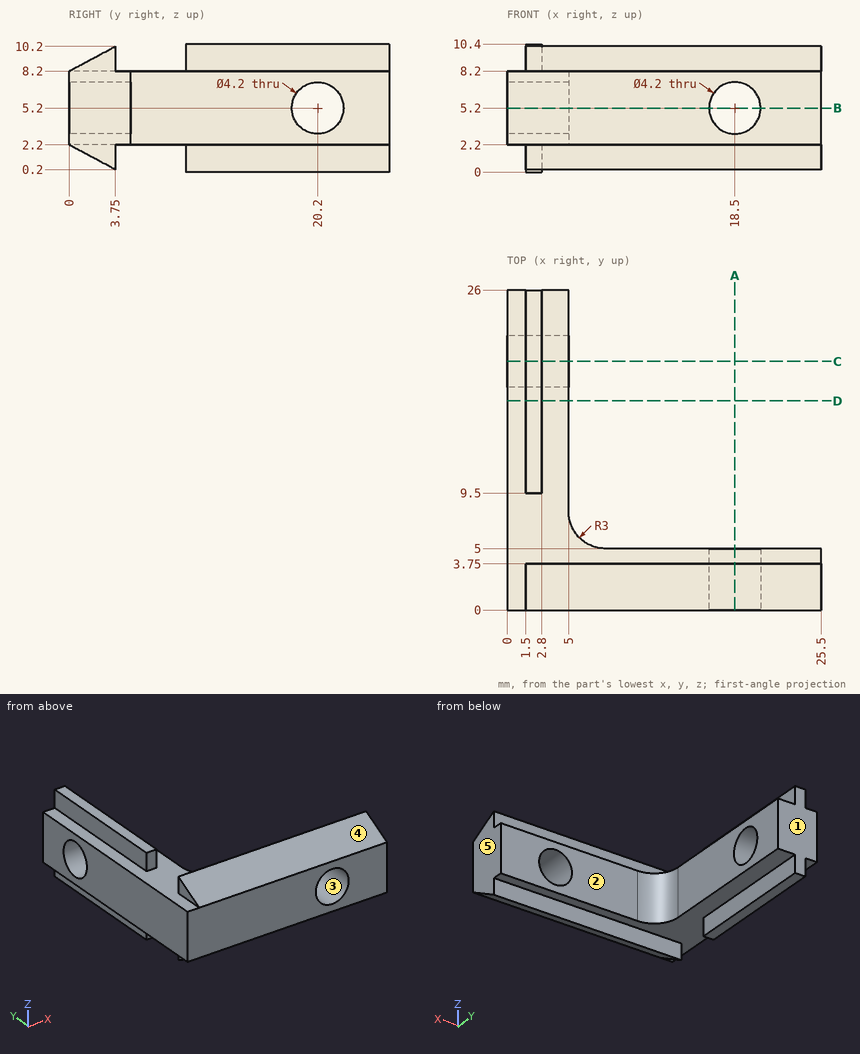
Study the drawing (mm; zero at the part's minimum x, y, z) and answer. A direction names the side the tool comes from. Coordinates: 2 decimals unless noted, no trailing zeros. Loops run counter-clockwise (first coordinate to the right, second up) from the corner with the lowest first, then second, coordinate; pieces in that order, holes last. Notation, with made-up numbers: (47.5, 27) -> (86.5, 27) arc R21 ccw to (86.5, 43) -> close; hole circle Ø8 at (0, -18.75). An arc over 180 degrees is marked (long way). Write each question's results on one line, items separated by ' | '. Start each with the question number.
1) For the marked faces 1 and 2, determine the directions among +Z, -Z, +X, -X, +Y, -Y from which every point of the face is accessible in a straight line to the end or side of a thin tool.
2) Find section D-D on y = 17. Determine the outline of the cut face in (x, z).
3) Find section A-A on x = 18.5. Determine the outline of the cut face in (y, z), then the cut area to 3 significant figures.
4) Consider line 1 along Z through (x, y) = (18.5, 3.9); line 2 along Y through (x, z) = (2.3, 5.2); line 3 along Z through (x, y) = (3.75, 11.25). Determine where each line is inside the solid, lowest interval first.
5) Find section C-C on y = 20.2. Determine the outline of the cut face in (x, z).
6) The mould has two halves that part along Z. Classify the marked faces 3, 4 and 5: pulls with the +Z half, pulls with the -Z half, needs draft (parallel to the pull), parting line crosses it, or undercut.
7) Flat-ended cylindrical pins translate along their axes: P1, Ø10, axis at x = 22.5, y = 6, coming from the -Z side; P2, Ø2.5, axis at y = 13.5, z = 0.5, coming from the +X side; P3, Ø2, axis at x = 6.5, z = 6.5, coming from the +Y side; P4, Ø3.5, axis at y = 20.2, z = 5.2, coming from the +X side. Find the tip coordinate at first contact, or state that the pin passes through.
8) Find section B-B on z = 5.2. Determine the outline of the cut face in (x, y).
Response values:
1) face 1: +Z, -Z, +X, -X, +Y | face 2: +Z, -Z, +X, +Y
2) outline: (0, 2.2) -> (1.5, 2.2) -> (1.5, 0) -> (2.8, 0) -> (2.8, 2.2) -> (5, 2.2) -> (5, 8.2) -> (2.8, 8.2) -> (2.8, 10.4) -> (1.5, 10.4) -> (1.5, 8.2) -> (0, 8.2) -> close
3) outline: (0, 2.2) -> (3.75, 0.2) -> (3.75, 2.2) -> (5, 2.2) -> (5, 3.1) -> (0, 3.1) -> close; (0, 7.3) -> (5, 7.3) -> (5, 8.2) -> (3.75, 8.2) -> (3.75, 10.2) -> (0, 8.2) -> close | area: 16.5 mm^2
4) line 1: z = 2.2 to 3.1, 7.3 to 8.2 | line 2: y = 0 to 18.1, 22.3 to 26 | line 3: z = 2.2 to 8.2
5) outline: (0, 2.2) -> (1.5, 2.2) -> (1.5, 0) -> (2.8, 0) -> (2.8, 2.2) -> (5, 2.2) -> (5, 3.1) -> (0, 3.1) -> close; (0, 7.3) -> (5, 7.3) -> (5, 8.2) -> (2.8, 8.2) -> (2.8, 10.4) -> (1.5, 10.4) -> (1.5, 8.2) -> (0, 8.2) -> close
6) face 3: undercut | face 4: pulls with the +Z half | face 5: needs draft
7) P1: stops at z = 0.2 | P2: stops at x = 2.8 | P3: stops at y = 6.34 | P4: passes through
8) outline: (0, 0) -> (16.4, 0) -> (16.4, 5) -> (8, 5) arc R3 cw to (5, 8) -> (5, 18.1) -> (0, 18.1) -> close; (0, 22.3) -> (5, 22.3) -> (5, 26) -> (0, 26) -> close; (20.6, 0) -> (25.5, 0) -> (25.5, 5) -> (20.6, 5) -> close
